```python
from build123d import *

# Parameters (mm, degrees)
BLANKSKE_W          = 55
BLANKSKE_H          = 9
BLANK_DEPTH         = 8
TOOTHCUTSIM_DEPTH   = 57.302753041
TEETHCUTS_COUNT     = 18
TEETHCUTS_PITCH     = 3.14159265
SKETCH1_W           = 8
SKETCH1_H           = 9
BOSS_EXTRUDE1_DEPTH = 8
SKETCH2_W           = 8.329556553
SKETCH2_H           = 8
BOSS_EXTRUDE2_DEPTH = 4
SKETCH3_W           = 8
SKETCH3_H           = 4
BOSS_EXTRUDE3_DEPTH = 5


with BuildPart() as part:
    # BlankSke → Blank (new body)
    with BuildSketch(Plane.XY):
        with Locations((27.5, 4.5)):
            Rectangle(BLANKSKE_W, BLANKSKE_H)
    extrude(amount=-BLANK_DEPTH)

    # TooCutSkeSim → ToothCutSim (cut, through all)
    with BuildSketch(Plane.XY):
        Polygon((0.44443537, 6.75), (-0.44443537, 6.75), (-1.272613241, 9.0254), (1.272613241, 9.0254), align=None)
    toothcutsim = extrude(amount=-TOOTHCUTSIM_DEPTH, mode=Mode.SUBTRACT)

    # TeethCuts: ToothCutSim ×18
    with Locations(*[(i * TEETHCUTS_PITCH, 0, 0) for i in range(1, TEETHCUTS_COUNT)]):
        add(toothcutsim, mode=Mode.SUBTRACT)

    # Sketch1 → Boss-Extrude1 (add)
    with BuildSketch(Plane(origin=(55, 0, 0), x_dir=(0, 0, -1), z_dir=(1, 0, 0))):
        with Locations((4, 4.5)):
            Rectangle(SKETCH1_W, SKETCH1_H)
    extrude(amount=BOSS_EXTRUDE1_DEPTH)

    # Sketch2 → Boss-Extrude2 (add)
    with BuildSketch(Plane(origin=(0, 9, 0), x_dir=(1, 0, 0), z_dir=(0, 1, 0))):
        with Locations((58.835221724, 4)):
            Rectangle(SKETCH2_W, SKETCH2_H)
    extrude(amount=BOSS_EXTRUDE2_DEPTH)

    # Sketch3 → Boss-Extrude3 (add)
    with BuildSketch(Plane(origin=(0, 0, -8), x_dir=(-1, 0, 0), z_dir=(0, 0, -1))):
        with Locations((-59, 11)):
            Rectangle(SKETCH3_W, SKETCH3_H)
    extrude(amount=BOSS_EXTRUDE3_DEPTH)


solid = part.part
```
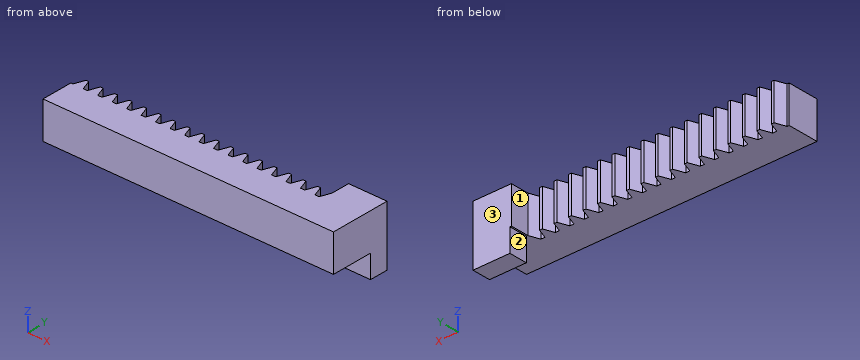
Work out the finished part from the listing and answer in its coordinate system (mm). Face numbers are marked on the shaded views. A direction names the side the tool comes from. Give positions to 0.01 mm unless a question says otherwise; leave off trailing zeros. Order: outer loops, then holes, each group sorted by start corner. A loop starts at its lowest first (then second) coordinate and runs counter-clockwise, first axis right, second up. Notation, with made-up numbers: (57.25, 14) -> (108.25, 14) arc R23 cw to (108.25, 29) -> close; hole circle Ø5 at (-28, -2.75). An arc over 180 degrees is marked (long way). Answer as CSV lines item,"result". Start each with the question number.
(1) Section B-B, the plane x = 56 is taken. Write down the section's boundary in (y, z).
(2) Which of the six approach directions +Z, -Z, +X, -X, +Y, -Y give full straight-line access (tool end or side, diameter ignored) to the marked faces 1, 2 and 3?
(3) Consider line 1 along Z through (x, y) = (27, 1); line 2 along Y through (x, z) = (14, -2.75); line 3 along X through (y, z) = (12, -10.75). Determine where each line is inside the solid, lowest interval first.
(4) Each of these flat-tipped pins is pushed along its axis until it touches: pin 1 Ø4 at (x, z) = (13.5, -11) entering from -Y; pin 2 Ø0.7 at (x, z) = (30, -5.5) entering from +Y; pin 3 Ø5 at (x, y) = (38, 3) entering from -Z; pin 4 Ø4.5 at (y, z) = (11.5, -4.5) entering from -X. Where does it stop, or does it pass through?
(5) Section C-C, the plane z = -9.25 is taken. Write down the section's boundary in (x, y).
(6) Section D-D, the plane y = 5 is taken. Write down the section's boundary in (x, z), plus the area to 3 significant figures.
(7) Section A-A, the plane y = 10.5 is taken. Write down the section's boundary in (x, z).
Entries:
1,outline,"(0, -8) -> (9, -8) -> (9, -13) -> (13, -13) -> (13, 0) -> (0, 0) -> close"
2,face 1,"+Z, -Z, -X, +Y"
2,face 2,"-Z, -X, +Y, -Y"
2,face 3,"+Z, -Z, +X, -X, +Y"
3,line 1,"-8 to 0"
3,line 2,"0 to 9"
3,line 3,"55 to 63"
4,pin 1,"through"
4,pin 2,"y = 9"
4,pin 3,"z = -8"
4,pin 4,"x = 54.67"
5,outline,"(55, 9) -> (63, 9) -> (63, 13) -> (55, 13) -> close"
6,outline,"(0, -8) -> (63, -8) -> (63, 0) -> (0, 0) -> close"
6,area,"504 mm²"
7,outline,"(54.67, -8) -> (55, -8) -> (55, -13) -> (63, -13) -> (63, 0) -> (54.67, 0) -> close"
